The listing builds one solid part. Answer for the finished solid, in the listing's coordinates (mm). Face numbers are marked on the shaded views. A direction names the side the tool comes from. Round coordinates to 2 decimals unless told otherwise and drop trailing zeros. Write each loop counter-clockwise with the first axis right and the second up, starting at its lowest first coordinate (ties: lowest second). Pieces come first, ordered by that corner, then holes.
Item 1: Find the intervals of material crossed by probe 1 along Y at (x, z) = (-15.2, 0); probe 2 along Y at (x, z) = (-7.5, 35.5); probe 3 along X at (y, z) = (58, 17), in increasing order.
Item 2: Find section B-B on z = -33. Give the vertices of the cut face in (x, y), then the cut area to 3 significant figures.
Item 3: A tool of negligible diameter and unlimited length cuts with its end or side. For the marked faces 1, 2 and 3, from which of +Z, -Z, +X, -X, +Y, -Y can it reach the whole face along a straight path? Write none if from no direction.
Item 4: Each of these flat-tipped pins is pushed along its axis until it touches: pin 1 (6 mm diameter, centred on x = 38.5, z = -17.5, fed in from +Y); pin 2 (3 mm diameter, centred on y = 88.5, z = -14.5, fed in from +X); pin 3 (9.5 mm diameter, centred on y = 88, z = 2, fed in from -X). Where does it stop, or does it pass through?
Item 5: Find section A-A on y = 119. Give the vertices of the cut face in (x, z), then the cut area to 3 significant figures.
Item 6: Find section C-C on x = -22. Give the vertices of the cut face in (y, z), then the cut area to 3 significant figures.
```python
from build123d import *

# Parameters (mm, degrees)
CUT_EXTRUDE1_DEPTH = 14
CIRPATTERN1_COUNT  = 4
CIRPATTERN2_COUNT  = 4
CHAMFER3_SIZE      = 2


with BuildPart() as part:
    # Sketch1 → Revolve1 (revolve)
    with BuildSketch(Plane.XY, mode=Mode.PRIVATE) as revolve1_sk:
        Polygon((7.5, 0), (7.5, 30), (6, 30), (6, 36), (20, 36), (20, 76), (18, 76), (18, 82), (50, 82), (50, 96), (14, 96), (14, 102), (16, 102), (16, 132), (8, 132), (8, 164), (0, 164), (0, 0), align=None)
    revolve(revolve1_sk.sketch.rotate(Axis((0, 0, 0), (0, 1, 0)), 90), axis=Axis((0, 0, 0), (0, 1, 0)))  # turned: the seam where the file's is

    # Sketch2 → Cut-Extrude1 (cut)
    with BuildSketch(Plane(origin=(0, 96, 0), x_dir=(1, 0, 0), z_dir=(0, 1, 0))):
        with BuildLine():
            Line((42, 6), (49.638694584, 6))
            ThreePointArc((49.638694584, 6), (50, 0), (49.638694584, -6))
            Line((49.638694584, -6), (42, -6))
            Line((42, -6), (42, 6))
        make_face()
    cut_extrude1 = extrude(amount=-CUT_EXTRUDE1_DEPTH, mode=Mode.SUBTRACT)

    # CirPattern1: Cut-Extrude1 ×4 about axis
    cirpattern1_axis = Axis((0, 0, 0), (0, 1, 0))
    for i in range(1, CIRPATTERN1_COUNT):
        add(cut_extrude1.rotate(cirpattern1_axis, i * 360 / CIRPATTERN1_COUNT), mode=Mode.SUBTRACT)

    # Sketch6 → CBORE for #12 Binding Head Machine Screw3 (revolve, cut)
    with BuildSketch(Plane(origin=(0, 58, 20), x_dir=(0, -1, 0), z_dir=(1, 0, 0))):
        Polygon((0, 0), (0, 9.739852008), (2.8956, 8), (2.8956, 3.5814), (5.95376, 3.5814), (5.95376, 0), align=None)
    cbore_for_12_binding_head_machine_screw = revolve(axis=Axis((0, 58, 26.35), (0, 0, -1)), mode=Mode.SUBTRACT)

    # CirPattern2: CBORE for #12 Binding Head Machine Screw3 ×4 about axis
    cirpattern2_axis = Axis((0, 0, 0), (0, 1, 0))
    for i in range(1, CIRPATTERN2_COUNT):
        add(cbore_for_12_binding_head_machine_screw.rotate(cirpattern2_axis, i * 360 / CIRPATTERN2_COUNT), mode=Mode.SUBTRACT)

    # Chamfer3
    chamfer3_edges = [part.edges().sort_by_distance(p)[0] for p in [
        (0, 36, 20),
    ]]
    chamfer(chamfer3_edges, length=CHAMFER3_SIZE)


solid = part.part
```
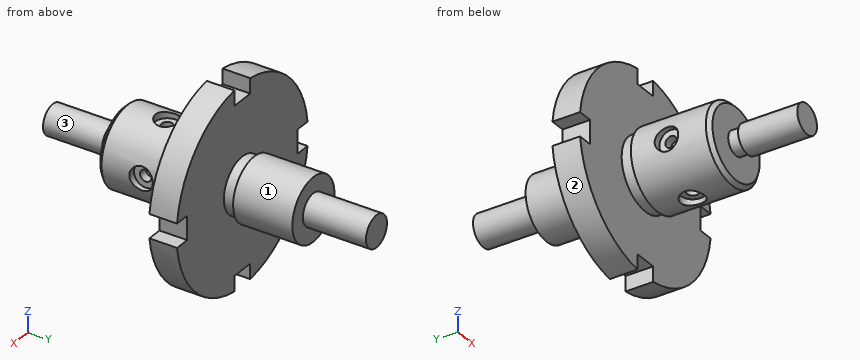
Check values:
1. probe 1: y = 36 to 55.1, 60.9 to 96, 102 to 132
1. probe 2: y = 82 to 96
1. probe 3: x = -10.54 to -5.95, 5.95 to 10.54
2. outline: (-37.56, 82) - (37.56, 82) - (37.56, 96) - (-37.56, 96) - close
2. area: 1,050 mm2
3. face 1: +Y
3. face 2: -Z, -X, +Y, -Y
3. face 3: -Y
4. pin 1: stops at y = 96
4. pin 2: stops at x = 48.28
4. pin 3: stops at x = -49.64
5. outline: circle Ø32 at (0, 0)
5. area: 804 mm2
6. outline: (82, -44.9) - (96, -44.9) - (96, 44.9) - (82, 44.9) - close
6. area: 1,260 mm2
